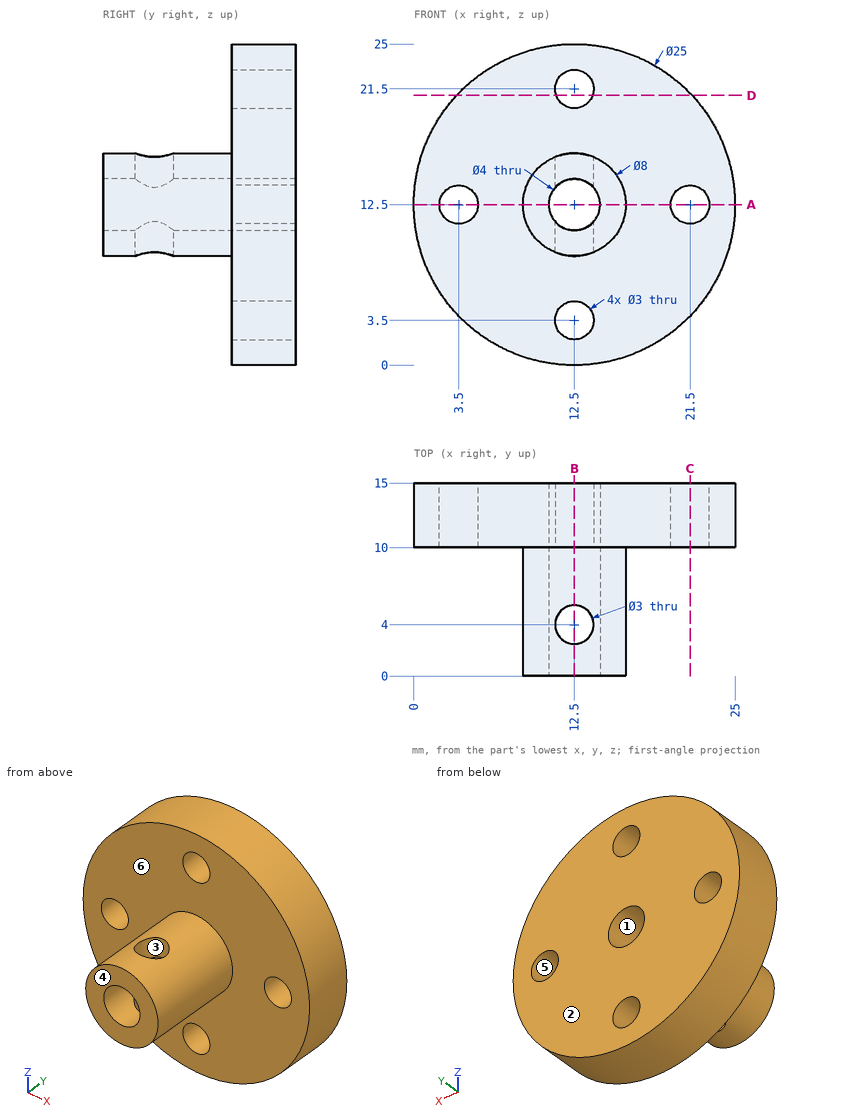
Study the drawing (mm; zero at the part's minimum x, y, z) and answer. A direction names the side the tool comes from. Coordinates: 2 decimals unless noted, no trailing zeros. Write each loop counter-clockwise with the first axis right and the second up, starting at its lowest first coordinate (ties: lowest second). Pieces come first, ordered by that corner, then holes. Notation, with made-up numbers: (14.25, 79) - (52.25, 79) arc R16 ccw to (52.25, 86) - close; hole circle Ø3 at (-10, 80.5). An arc over 180 degrees is marked (long way). Answer as a JSON object with one key per item and string values.
Q1. Which of the six approach directions +Z, -Z, +X, -X, +Y, -Y give full straight-line access (tool end or side, diameter ignored) to the marked faces 5 and 6?
Results list:
{"face 5": "+Y, -Y", "face 6": "-Y"}
Q2. Consider L1, parallel to X at y = 11.9, z = 12.5; L2, parallel to Y at x = 12.5, z = 14.7; L3, parallel to Y at x = 12.5, z = 23.5. Determine where each line is inside the solid, lowest interval first. Write a range as from..to.
Results list:
{"L1": "x = 0..2, 5..10.5, 14.5..20, 23..25", "L2": "y = 0..2.5, 5.5..15", "L3": "y = 10..15"}
Q3. Find section D-D (z = 21). Write down the section's boundary in (x, y).
Results list:
{"outline": "(3.33, 10) - (11.09, 10) - (11.09, 15) - (3.33, 15) - close; (13.91, 10) - (21.67, 10) - (21.67, 15) - (13.91, 15) - close"}
Q4. Find section C-C (x = 21.5). Write down the section's boundary in (y, z).
Results list:
{"outline": "(10, 3.83) - (15, 3.83) - (15, 11) - (10, 11) - close; (10, 14) - (15, 14) - (15, 21.17) - (10, 21.17) - close"}
Q5. For a pull along Y with two mould halves and no side action, classify the marked faces 1, 2, 3 and 4 as pulls with the +Y half, pulls with the -Y half, needs draft (parallel to the pull), parting line crosses it, or undercut.
Results list:
{"face 1": "needs draft", "face 2": "pulls with the +Y half", "face 3": "undercut", "face 4": "pulls with the -Y half"}
Q6. Given pin 1 Ø5 at (x, z) = (12.5, 21.5) entering from -Y; pin 2 Ø3 at (x, z) = (12.5, 12.5) entering from +Y; pin 3 Ø4 at (x, y) = (12.5, 4) entering from -Z; pin 4 Ø2 at (y, z) = (6, 17) entering from -X, each flat-ended and moving along its own axis, determine where each tip first touches the part or whether it passes through.
Results list:
{"pin 1": "stops at y = 10", "pin 2": "passes through", "pin 3": "stops at z = 8.5", "pin 4": "stops at x = 10.56"}
Q7. Find section A-A (z = 12.5). Write down the section's boundary in (x, y), plus the area to 3 significant figures.
Results list:
{"outline": "(0, 10) - (2, 10) - (2, 15) - (0, 15) - close; (5, 10) - (8.5, 10) - (8.5, 0) - (10.5, 0) - (10.5, 15) - (5, 15) - close; (14.5, 0) - (16.5, 0) - (16.5, 10) - (20, 10) - (20, 15) - (14.5, 15) - close; (23, 10) - (25, 10) - (25, 15) - (23, 15) - close", "area": "115 mm^2"}
Q8. Find section B-B (x = 12.5). Write down the section's boundary in (y, z), plus the area to 3 significant figures.
Results list:
{"outline": "(0, 8.5) - (2.5, 8.5) - (2.5, 10.5) - (0, 10.5) - close; (0, 14.5) - (2.5, 14.5) - (2.5, 16.5) - (0, 16.5) - close; (5.5, 8.5) - (10, 8.5) - (10, 5) - (15, 5) - (15, 10.5) - (5.5, 10.5) - close; (5.5, 14.5) - (15, 14.5) - (15, 20) - (10, 20) - (10, 16.5) - (5.5, 16.5) - close; (10, 0) - (15, 0) - (15, 2) - (10, 2) - close; (10, 23) - (15, 23) - (15, 25) - (10, 25) - close", "area": "103 mm^2"}
